Autodesk Inventor part; units mm, degrees
ref_plane "YZ Plane" through (0, 0, 0) normal (1, 0, 0) x (0, 1, 0)
ref_plane "XZ Plane" through (0, 0, 0) normal (0, 1, 0) x (-1, 0, 0)
ref_plane "XY Plane" through (0, 0, 0) normal (0, 0, 1) x (1, 0, 0)
sketch "Sketch3" plane through (0, 0, 0) normal (0, 1, 0) x (-1, 0, 0)
  circle A0 centre (0, 0) radius 95
  line L0 (-68, 0) -> (-68, -40)
  line L1 (-68, 0) -> (-68, 40)
  line L2 (-68, 40) -> (-86.1684, 40)
  line L3 (-68, -40) -> (-86.1684, -40)
  line L4 (-56, 0) -> (-56, -76.7398)
  line L5 (-56, 0) -> (-56, 76.7398)
  line L6 (-62, 0) -> (-62, -15)
  line L7 (-62, 0) -> (-62, 15)
  circle A1 centre (-62, 15) radius 1.5
  circle A2 centre (-62, 0) radius 1.5
  circle A3 centre (-62, -15) radius 1.5
  line L8 (-68, 0) -> (-70, 0)
  line L9 (-70, 0) -> (-70, -40)
  line L10 (-70, 0) -> (-70, 40)
  dimension "d1" = 68
  dimension "d2" = 40
  dimension "d3" = 40
  dimension "d4" = 12
  dimension "d5" = 6
  dimension "d6" = 15
  dimension "d7" = 15
  dimension "d8" = 3
  dimension "d9" = 3
  dimension "d10" = 3
  dimension "d11" = 2
extrude "Extrusion1" add sketch "Sketch3" along normal blind 2 contours L5 L4 A0 L3 L0 L1 L2 | L2 L1 L8 L10 | L9 L8 L0 L3
sketch "Sketch4" plane through (0, 0, 0) normal (0, -1, 0) x (1, 0, 0)
  line L0 (70, 40) -> (70, -40)
  line L1 (70, 0) -> (68, 0)
  line L2 (68, 0) -> (68, -40)
  line L3 (70, -41) -> (85.6971, -41)
  arc A0 (56, -76.7398) -> (86.1684, -40) centre (0, 0) ccw
  line L4 (68, -40) -> (68, -41)
  line L5 (70, -41) -> (68, -41)
  line L6 (85.6971, -41) -> (86.1684, -40)
  line L7 (70, -40) -> (86.1684, -40)
  line L8 (70, -40) -> (86.1684, -40)
  line L9 (70, -40) -> (70, 40)
  line L10 (86.1684, 40) -> (70, 40)
  line L11 (86.1684, 40) -> (70, 40)
  line L12 (68, 0) -> (68, 40)
  line L13 (70, 41) -> (85.6971, 41)
  arc A1 (86.1684, 40) -> (56, 76.7398) centre (0, 0) ccw
  line L14 (70, 41) -> (68, 41)
  line L15 (68, 40) -> (68, 41)
  line L16 (85.6971, 41) -> (86.1684, 40)
  dimension "d14" = 2
  dimension "d15" = 1
extrude "Extrusion2" add sketch "Sketch4" along normal blind 39.5
sketch "Sketch5" plane through (0, -39.5, 0) normal (0, -1, 0) x (1, 0, 0)
  point P0 (0, 0)
sketch "Sketch6" plane through (0, -39.5, 0) normal (0, -1, 0) x (1, 0, 0)
  circle A0 centre (62, 15) radius 1.5
  circle A1 centre (62, 15) radius 1.5
  circle A2 centre (62, 0) radius 1.5
  circle A3 centre (62, -15) radius 1.5
  circle A4 centre (62, -15) radius 1.5
  line L0 (70, 40) -> (56, 40)
  line L1 (70, -40) -> (86.1684, -40)
  line L2 (70, -40) -> (56, -40)
  line L3 (56, -40) -> (56, 40)
  line L4 (70, 40) -> (70, -40)
  line L5 (70, 40) -> (70, -40)
  line L6 (86.1684, 40) -> (70, 40)
  line L7 (86.1684, 40) -> (70, 40)
  line L8 (70, -40) -> (86.1684, -40)
  line L9 (86.1684, 40) -> (85.6971, 41)
  arc A5 (86.1684, 40) -> (85.6971, 41) centre (0, 0) ccw
  line L10 (56, 40) -> (56, 41)
  line L11 (85.6971, 41) -> (56, 41)
  line L12 (56, -40) -> (56, -41)
  line L13 (86.1684, -40) -> (85.9357, -40.5014)
  line L14 (85.6971, -41) -> (56, -41)
  line L15 (85.9357, -40.5014) -> (85.6971, -41)
  arc A6 (56, -76.7398) -> (86.1684, -40) centre (0, 0) ccw
extrude "Extrusion3" add sketch "Sketch6" along normal blind 2 contours L4 L2 L3 L0
extrude "Extrusion5" add sketch "Sketch6" along normal blind 2 contours L0 L10 L11 L9 L6 | L1 L13 L15 L14 L12 L2
sketch "Sketch7" plane through (70, 2, 40) normal (1, 0, 0) x (0, 0, -1)
  line L0 (0, -2) -> (0, -43.5)
  line L1 (80, -2) -> (80, -41.5)
  line L2 (80, -21.75) -> (55, -21.75)
  line L3 (55, -21.75) -> (40, -21.75)
  line L4 (40, -21.75) -> (40, -3.75)
  line L5 (40, -21.75) -> (40, -39.75)
  line L6 (55, -21.75) -> (55, -3.75)
  line L7 (55, -21.75) -> (55, -39.75)
  line L8 (0, 0) -> (80, 0)
  line L9 (0, -22.5) -> (25, -22.5)
  line L10 (25, -22.5) -> (25, -4.5)
  line L11 (25, -22.5) -> (25, -40.5)
  line L12 (25, -4.5) -> (25, -40.5) construction
  line L13 (23.5, -4.5) -> (23.5, -40.5)
  line L14 (26.5, -40.5) -> (26.5, -4.5)
  arc A0 (26.5, -4.5) -> (23.5, -4.5) centre (25, -4.5) ccw
  arc A1 (23.5, -40.5) -> (26.5, -40.5) centre (25, -40.5) ccw
  line L15 (40, -3.75) -> (40, -39.75) construction
  line L16 (38.5, -3.75) -> (38.5, -39.75)
  line L17 (41.5, -39.75) -> (41.5, -3.75)
  arc A2 (41.5, -3.75) -> (38.5, -3.75) centre (40, -3.75) ccw
  arc A3 (38.5, -39.75) -> (41.5, -39.75) centre (40, -39.75) ccw
  line L18 (55, -39.75) -> (55, -3.75) construction
  line L19 (56.5, -39.75) -> (56.5, -3.75)
  line L20 (53.5, -3.75) -> (53.5, -39.75)
  arc A4 (53.5, -39.75) -> (56.5, -39.75) centre (55, -39.75) ccw
  arc A5 (56.5, -3.75) -> (53.5, -3.75) centre (55, -3.75) ccw
  point P0 (40, -2)
  point P1 (40, -21.75)
  dimension "d26" = 25
  dimension "d27" = 15
  dimension "d28" = 18
  dimension "d29" = 18
  dimension "d30" = 18
  dimension "d31" = 18
  dimension "d35" = 21.75
  dimension "d36" = 25
  dimension "d37" = 18
  dimension "d38" = 18
  dimension "d39" = 3
  dimension "d40" = 3
  dimension "d41" = 3
extrude "Extrusion6" cut sketch "Sketch7" against normal blind 2
properties part number "Base-Dribler"
Read the model definition and answer for the solid it produces. Units are mm, in the model's axes. A direction names the side the tool comes from. Round coordinates to 2 decimals unless told otherwise and drop trailing zeros. Order: outer loops, then holes, each group sorted by start corner. A loop starts at its lowest first (then second) coordinate and runs counter-clockwise, first axis right, second up.
1) The part is cut by section D-D on x = 74. Write down the section's boundary in (y, z).
2) The mould has two halves that part along Y. Classify faces 1 (the face through (64, -41.5, 1)), 2 (the face through (63.43, -40.49, 14.55)), 3 (the face through (59, -39.5, 1)): released by +Y, released by -Y, zero draft, split by the parting line, or undercut.
3) The part is cut by section C-C on x = 83.5. Write down the section's boundary in (y, z).
4) For faces 4 (the face through (78, -20, -41)), 5 (the face through (68, -19, -10)), 6 (the face through (78, -20, 41)), 7 (the face through (78, -19, -40)), determine the directions among +Z, -Z, +X, -X, +Y, -Y from which every point of the face is accessible in a straight line to the end or side of a thin tool.
5) Straight lines are drawn through the part: L1, parallel to Z at x = 62, y = -40.5; L2, parallel to Z at x = 73, y = -28; L3, parallel to Y at x = 58.5, z = -16. For each, find the intervals that lie inside material, in ascending order.
6) Flat-ended cylindrical pins translate along their axes: pin 1 (1 mm diameter, centred on x = 69, y = -13.5, fed in from -Z); pin 2 (5 mm diameter, centred on x = 65, y = -19.5, fed in from +Z); pin 3 (3 mm diameter, centred on y = -4, z = -32.5, fed in from -X); pin 4 (1 mm diameter, centred on x = 69.5, y = -24.5, fed in from +Z). Find the tip coordinate at first contact, or state that the pin passes through.
7) The part is cut by section A-A on y = -21.5. Write down the section's boundary in (x, z).
8) The part is cut by section B-B on z = -15. Write down the section's boundary in (x, y), plus the area to 3 significant figures.
Resolved:
1. outline: (-41.5, -41) - (0, -41) - (0, -59.57) - (2, -59.57) - (2, -40) - (-41.5, -40) - close; (-41.5, 40) - (2, 40) - (2, 59.57) - (0, 59.57) - (0, 41) - (-41.5, 41) - close
2. face 1: released by -Y
2. face 2: zero draft
2. face 3: undercut
3. outline: (-41.5, -41) - (0, -41) - (0, -45.31) - (2, -45.31) - (2, -40) - (-41.5, -40) - close; (-41.5, 40) - (2, 40) - (2, 45.31) - (0, 45.31) - (0, 41) - (-41.5, 41) - close
4. face 4: -Z, +X, -X, -Y
4. face 5: +Z, -Z, -X
4. face 6: +Z, +X, -X, -Y
4. face 7: +X, +Y, -Y
5. L1: z = -41 to -16.5, -13.5 to -1.5, 1.5 to 13.5, 16.5 to 41
5. L2: z = -41 to -40, 40 to 41
5. L3: y = -41.5 to -39.5, 0 to 2
6. pin 1: stops at z = -41
6. pin 2: passes through
6. pin 3: stops at x = 68
6. pin 4: stops at z = 41
7. outline: (68, -41) - (85.7, -41) arc R95 ccw to (86.17, -40) - (70, -40) - (70, -16.5) - (68, -16.5) - close; (68, -13.5) - (70, -13.5) - (70, -1.5) - (68, -1.5) - close; (68, 1.5) - (70, 1.5) - (70, 13.5) - (68, 13.5) - close; (68, 16.5) - (70, 16.5) - (70, 40) - (86.17, 40) arc R95 ccw to (85.7, 41) - (68, 41) - close
8. outline: (56, -41.5) - (60.5, -41.5) - (60.5, -39.5) - (56, -39.5) - close; (56, 0) - (60.5, 0) - (60.5, 2) - (56, 2) - close; (63.5, -41.5) - (70, -41.5) - (70, -39.25) - (68, -39.25) - (68, -39.5) - (63.5, -39.5) - close; (63.5, 0) - (68, 0) - (68, -0.25) - (70, -0.25) - (70, 2) - (63.5, 2) - close
8. area: 45.0 mm2
